```python
from build123d import *

# Parameters (mm, degrees)
SKETCH006_R     = 3
PAD005_DEPTH    = 1
SKETCH012_R     = 0.5
POCKET002_DEPTH = 2
POCKET003_DEPTH = 5
CHAMFER_SIZE    = 0.5


with BuildPart() as part:
    # Sketch006 (on ShapeBinder) → Pad005 (new body)
    with BuildSketch(Plane(origin=(0, 0, 0), x_dir=(1, 0, 0), z_dir=(0, 0, -1))):
        with BuildLine():
            ThreePointArc((-7.987387, 2.907171), (-8.333808, 1.672617), (-8.490583, 0.4))
            Line((-7.689603, 0.4), (-8.490583, 0.4))
            ThreePointArc((-7.689603, 0.4), (-7.7, 0), (-7.689603, -0.4))
            Line((-7.689603, -0.4), (-8.490583, -0.4))
            ThreePointArc((-8.490583, -0.4), (-8.333808, -1.672617), (-7.987387, -2.907171))
            Line((-7.987387, -2.907171), (-7.496671, -2.792834))
            ThreePointArc((-7.496671, -2.792834), (-7.082093, -3.720747), (-6.553216, -4.588611))
            Line((-6.962792, -4.8754), (-6.553216, -4.588611))
            ThreePointArc((-6.962792, -4.8754), (0, -8.5), (6.962792, -4.8754))
            Line((6.962792, -4.8754), (6.553216, -4.588611))
            ThreePointArc((6.553216, -4.588611), (7.082093, -3.720747), (7.496671, -2.792834))
            Line((7.987387, -2.907171), (7.496671, -2.792834))
            ThreePointArc((7.987387, -2.907171), (8.333808, -1.672617), (8.490583, -0.4))
            Line((8.490583, -0.4), (7.689603, -0.4))
            ThreePointArc((7.689603, -0.4), (7.7, 0), (7.689603, 0.4))
            Line((8.490583, 0.4), (7.689603, 0.4))
            ThreePointArc((8.490583, 0.4), (8.333808, 1.672617), (7.987387, 2.907171))
            Line((7.987387, 2.907171), (7.496671, 2.792834))
            ThreePointArc((7.496671, 2.792834), (7.082093, 3.720747), (6.553216, 4.588611))
            Line((6.962792, 4.8754), (6.553216, 4.588611))
            Line((6.962792, 4.8754), (6.962792, 11.5))
            Line((6.962792, 11.5), (-6.962792, 11.5))
            Line((-6.962792, 4.8754), (-6.962792, 11.5))
            Line((-6.962792, 4.8754), (-6.553216, 4.588611))
            ThreePointArc((-6.553216, 4.588611), (-7.082093, 3.720747), (-7.496671, 2.792834))
            Line((-7.987387, 2.907171), (-7.496671, 2.792834))
        make_face()
        Circle(SKETCH006_R, mode=Mode.SUBTRACT)
    extrude(amount=PAD005_DEPTH)

    # Sketch012 (on Face28 of Pad005) → Pocket002 (cut)
    with BuildSketch(Plane.XY):
        with Locations((0, -8.25)):
            Circle(SKETCH012_R)
        with Locations((-5, -8.25)):
            Circle(SKETCH012_R)
        with Locations((5, -8.25)):
            Circle(SKETCH012_R)
    extrude(amount=-POCKET002_DEPTH, mode=Mode.SUBTRACT)

    # Sketch013 (on Face4 of Pocket002) → Pocket003 (cut)
    with BuildSketch(Plane.XY):
        Polygon((-6.962792, -11.5), (-5.75, -11.5), (-5.75, -10.5), (-4.25, -10.5), (-4.25, -11.5), (-0.75, -11.5), (-0.75, -10.5), (0.75, -10.5), (0.75, -11.5), (4.25, -11.5), (4.25, -10.5), (5.75, -10.5), (5.75, -11.5), (6.962792, -11.5), (6.962792, -12.871278), (-6.962792, -12.871278), align=None)
    extrude(amount=-POCKET003_DEPTH, mode=Mode.SUBTRACT)

    # Chamfer
    chamfer_edges = [part.edges().sort_by_distance(p)[0] for p in [
        (-6.962792, -11.5, -0.5),
        (6.962792, -11.5, -0.5),
    ]]
    chamfer(chamfer_edges, length=CHAMFER_SIZE)


solid = part.part
```
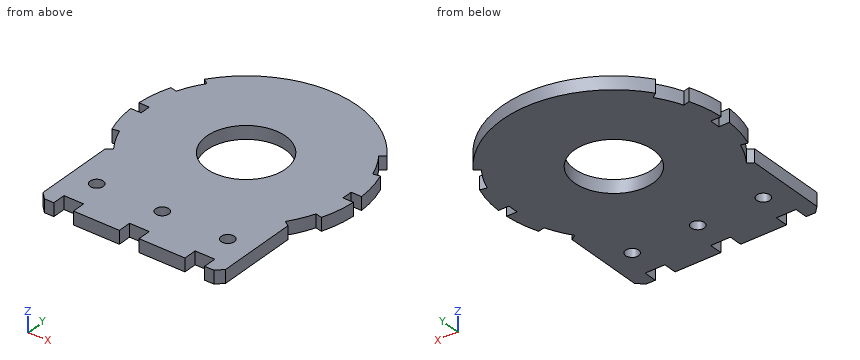
Model file for the job. Use its own axes, mm. Give positions to 0.01 mm unless a question says otherwise; leave off trailing zeros. Write each loop counter-clockwise with the first axis right and the second up, starting at its lowest first coordinate (ties: lowest second). Pieces come first, ordered by that corner, then holes. Notation, with made-up numbers: M 28.5,44 L 71.5,44 A27 ccw 71.5,73 Z; hole C 70,-16.75 d7. An arc over 180 degrees is marked long. Use a Markdown table: item, result.
1) Cut at A-A (x = 0). List the corners of the cut face in (y, z).
Responses:
| item | result |
|---|---|
| outline | M -10.5,-1 L -8.75,-1 L -8.75,0 L -10.5,0 Z; M -7.75,-1 L -3,-1 L -3,0 L -7.75,0 Z; M 3,-1 L 8.5,-1 L 8.5,0 L 3,0 Z |
2) Cut at C-C (y = -8.25). List the corners of the cut face in (x, z).
Responses:
| item | result |
|---|---|
| outline | M -6.96,-1 L -5.5,-1 L -5.5,0 L -6.96,0 Z; M -4.5,-1 L -0.5,-1 L -0.5,0 L -4.5,0 Z; M 0.5,-1 L 4.5,-1 L 4.5,0 L 0.5,0 Z; M 5.5,-1 L 6.96,-1 L 6.96,0 L 5.5,0 Z |
3) Drill centre lines: line 1 (X direction, y = 0, z = -0.2); line 2 (X direction, y = 1, z = -0.1); line 3 (Y direction, x = 5, z = -0.65). Where is each one in solid material? Low to high. Write a range as from..to.
Responses:
| item | result |
|---|---|
| line 1 | x = -7.7..-3, 3..7.7 |
| line 2 | x = -8.44..-2.83, 2.83..8.44 |
| line 3 | y = -10.5..-8.75, -7.75..6.87 |
4) Cut at B-B (y = 0). List the corners of the cut face in (x, z).
Responses:
| item | result |
|---|---|
| outline | M -7.7,-1 L -3,-1 L -3,0 L -7.7,0 Z; M 3,-1 L 7.7,-1 L 7.7,0 L 3,0 Z |
5) Cut at D-D (x = -5). List the corners of the cut face in (y, z).
Responses:
| item | result |
|---|---|
| outline | M -10.5,-1 L -8.75,-1 L -8.75,0 L -10.5,0 Z; M -7.75,-1 L 6.87,-1 L 6.87,0 L -7.75,0 Z |
6) Pin check, flat tips, straight feed: pin 1 (0.5 mm diameter, centred on y = -11, z = -0.5, fed in from -X); pin 2 (5.5 mm diameter, centred on x = 0, y = 0, fed in from +Z); pin 3 (0.6 mm diameter, centred on x = 8, z = -0.5, fed in from +Y). Stop position of each tip, or through.
Responses:
| item | result |
|---|---|
| pin 1 | stops at x = -6.96 |
| pin 2 | passes through |
| pin 3 | stops at y = 2.91 |
